from build123d import *

# Parameters (mm, degrees)
SKETCH1_W           = 9.525
SKETCH1_H           = 9.525
SKETCH1_W_2         = 6.35
BOSS_EXTRUDE1_DEPTH = 3.175
FILLET1_R           = 2.54


with BuildPart() as part:
    # Sketch1 → Boss-Extrude1 (new body)
    with BuildSketch(Plane.XY):
        with Locations((4.7625, -4.7625)):
            Rectangle(SKETCH1_W, SKETCH1_H)
        Polygon((28.575, 0), (0, 16.497783942), (0, 0), align=None)
        with Locations((19.05, -4.7625)):
            Rectangle(SKETCH1_W_2, SKETCH1_H)
    extrude(amount=BOSS_EXTRUDE1_DEPTH)

    # Fillet1
    # the kernel refuses this fillet: 2.54 mm, written as the material it takes off along each edge
    with BuildSketch(Plane(origin=(28.575, 0, -19.896514347), x_dir=(-0.8660254037844417, 0.4999999999999948, 0), z_dir=(0, 0, 1))) as fillet1_piece_1:
        with BuildLine():
            CenterArc((7.958605739, 2.54), FILLET1_R, 165.522487814, 104.477512186)
            Line((5.499261314, 3.175), (5.450074426, 3.1877))
            ThreePointArc((5.450074426, 3.1877), (2.724230657, 1.631494091), (-0.0254, 0.043994091))
            Line((-0.0254, 0.043994091), (0, -0.0508))
            Line((0, -0.0508), (7.958605739, -0.0508))
            Line((7.958605739, -0.0508), (7.958605739, 0))
        make_face()
    extrude(amount=42.968028694, mode=Mode.SUBTRACT)
    with BuildSketch(Plane(origin=(0, 16.497783942, -10.998522628), x_dir=(0, -1, 0), z_dir=(0, 0, 1))) as fillet1_piece_2:
        with BuildLine():
            CenterArc((FILLET1_R * 1.73205080757, FILLET1_R), FILLET1_R, 150, 120)
            Line((FILLET1_R * 0.866025403784, FILLET1_R * 1.5), (FILLET1_R * 0.848704895709, FILLET1_R * 1.51))
            Line((FILLET1_R * 0.848704895709, FILLET1_R * 1.51), (-FILLET1_R * 0.0346410161514, -FILLET1_R * 0.02))
            Line((-FILLET1_R * 0.0346410161514, -FILLET1_R * 0.02), (FILLET1_R * 1.73205080757, -FILLET1_R * 0.02))
            Line((FILLET1_R * 1.73205080757, -FILLET1_R * 0.02), (FILLET1_R * 1.73205080757, 0))
        make_face()
    extrude(amount=25.172045256, mode=Mode.SUBTRACT)


solid = part.part
Model file for the job. Use its own axes, mm. A direction names the side the tool comes from. Give positions to 0.01 mm unless a question says otherwise; leave off trailing zeros. Loops run counter-clockwise (first coordinate to the right, second up) from the corner with the lowest first, then second, coordinate; pieces in that order, holes last. Notation, with made-up numbers: (71.25, -3) -> (102.25, -3) arc R34 ccw to (102.25, 32) -> close; hole circle Ø10 at (37.25, -35.75). An arc over 180 degrees is marked (long way). Use a Markdown table: item, result. Add a question column.
(1) Slice it at A-A on y = -5.5. List the corners of the cut face in (x, z) (3 decimals).
(2) Tool access for faces 4 (the flat face through (22.225, -5, 2)), 5 (the flat face through (13, 0, 2)), 6 (the flat face through (5, -9.525, 2)): list every direction of +Z, -Z, +X, -X, +Y, -Y with a clear straight run to the whole face (end or side of a thin tool).
(3) Wall check: line 1 along X through (y, z) = (-3.5, 0.6) (3 decimals); line 2 along X through (y, z) = (2.75, 3); line 3 along Y through (x, z) = (21.5, 2.8) (3 decimals). Give the ranges that are in metal, low to high.
(4) Slice it at B-B on z = 1.7. List the corners of the cut face in (x, y) (3 decimals).
(5) Slice it at C-C on x = 12.25. List the corners of the cut face in (y, z) (3 decimals).
(6) Mould opens along X. For faces 1 (the flat face through (19, -9.525, 2)), 2 (the flat face through (9.525, -5, 2)), 3 (the cylindrical face through (1.302, 14.316, 1.565)) say: +X half, -X half, draft (parallel to the pull), parting line (faces both ways), or undercut.
(7) Drop a flat-ended pin along its axis: pin 1 Ø1.5 at (y, z) = (-2.5, 2) entering from +X (3 decimals). Give the stop position or say it passes through.
(8) Slice it at D-D on y = 4.5. List the corners of the cut face in (x, z) (3 decimals), and give its area (3 significant figures).
Filled sheet:
| question | item | result |
|---|---|---|
| 1 | outline | (0, 0) -> (9.525, 0) -> (9.525, 3.175) -> (0, 3.175) -> close; (15.875, 0) -> (22.225, 0) -> (22.225, 3.175) -> (15.875, 3.175) -> close |
| 2 | face 4 | +Z, -Z, +X, -Y |
| 2 | face 5 | +Z, -Z, -Y |
| 2 | face 6 | +Z, -Z, +X, -X, -Y |
| 3 | line 1 | 0 to 9.525, 15.875 to 22.225 |
| 3 | line 2 | 0 to 22.76 |
| 3 | line 3 | -9.525 to 4.085 |
| 4 | outline | (0, -9.525) -> (9.525, -9.525) -> (9.525, 0) -> (15.875, 0) -> (15.875, -9.525) -> (22.225, -9.525) -> (22.225, 0) arc R2.54 ccw to (21.683, 3.979) -> (3.81, 14.298) arc R2.54 ccw to (0, 12.098) -> close |
| 5 | outline | (0, 0) -> (9.425, 0) -> (9.425, 3.175) -> (0, 3.175) -> close |
| 6 | face 1 | draft |
| 6 | face 2 | undercut |
| 6 | face 3 | parting line |
| 7 | pin 1 | x = 22.225 |
| 8 | outline | (0, 0) -> (20.781, 0) -> (20.781, 3.175) -> (0, 3.175) -> close |
| 8 | area | 66.0 mm2 |
